For this review, take the finished solid that the model builds, in its own axes (mm). Round coordinates to 2 decimals unless told otherwise and drop trailing zeros. Loops run counter-clockwise (first coordinate to the right, second up) from the corner with the lowest first, then second, coordinate; pieces in that order, holes last. Notation, with made-up numbers: M -32.75,82 L -16.75,82 A28 ccw -16.75,111 Z; hole C 22,81.5 d3. An arc over 180 degrees is marked long. One line per question, with ' | ' between items. Start each with the question number.
1) We need section A-A (x = 25). Give the boundary of the cut face in (y, z).
2) For probe 1 along Y at (x, z) = (25, -0.95); probe 2 along X at (y, z) = (6, -1.15); probe 3 along Y at (x, z) = (-26.5, 1.4), list the stretches that pass through material, from the lowest coordinate up. Write a range as from..to.
3) For pin 1 Ø5.5 at (x, y) = (-11.42, 31.36) entering from +Z, flat-tipped, find the tip position at first contact; note if it passes through.
4) We need section B-B (z = 1.4). State how many separate pieces and enclosed holes the cut face has, and give its area (3 significant figures).
```python
from build123d import *

# Parameters (mm, degrees)
SKETCH1_W             = 330
SKETCH1_H             = 90
SKETCH1_R             = 19.05
BOSS_EXTRUDE1_DEPTH   = 2.5
M6_CLEARANCE_HOLE1_D  = 6.4
SKETCH3_R             = 8
CUT_EXTRUDE2_DEPTH    = 6
M5X0_8_TAPPED_HOLE1_D = 4.2
M5X0_8_TAPPED_HOLE3_D = 4.2
FILLET1_R             = 1.5
M3X0_5_TAPPED_HOLE1_D = 2.5


with BuildPart() as part:
    # Sketch1 → Boss-Extrude1 (new body, symmetric)
    with BuildSketch(Plane.XY):
        Rectangle(SKETCH1_W, SKETCH1_H)
        Circle(SKETCH1_R, mode=Mode.SUBTRACT)
    extrude(amount=BOSS_EXTRUDE1_DEPTH, both=True)

    # M6 Clearance Hole1 (through all)
    with Locations(Plane.XY.offset(2.5)):
        with Locations((-150, 30), (-25, 30), (-25, -30), (-150, -30)):
            m6_clearance_hole1 = Hole(M6_CLEARANCE_HOLE1_D / 2)

    # Mirror2: M6 Clearance Hole1 across plane
    add(m6_clearance_hole1.mirror(Plane(origin=(0, 0, 0), x_dir=(0, 0, 1), z_dir=(1, 0, 0))), mode=Mode.SUBTRACT)

    # Sketch3 → Cut-Extrude2 (cut, through all)
    with BuildSketch(Plane.XY.offset(2.5)):
        with Locations((-75, -0.6)):
            Circle(SKETCH3_R)
    cut_extrude2 = extrude(amount=-CUT_EXTRUDE2_DEPTH, mode=Mode.SUBTRACT)

    # M5x0.8 Tapped Hole1 (through all)
    with Locations(Plane.XY.offset(2.5)):
        with Locations((-95, -0.6), (-55, -0.6)):
            m5x0_8_tapped_hole1 = Hole(M5X0_8_TAPPED_HOLE1_D / 2)

    # Mirror1: Cut-Extrude2, M5x0.8 Tapped Hole1 across plane
    add(cut_extrude2.mirror(Plane(origin=(0, 0, 0), x_dir=(0, 0, 1), z_dir=(1, 0, 0))), mode=Mode.SUBTRACT)
    add(m5x0_8_tapped_hole1.mirror(Plane(origin=(0, 0, 0), x_dir=(0, 0, 1), z_dir=(1, 0, 0))), mode=Mode.SUBTRACT)

    # M5x0.8 Tapped Hole3 (through all)
    with Locations(Plane.XY.offset(2.5)):
        with Locations((-11.415072797, 31.362654751), (11.415072797, -31.362654751), (-31.362654751, -11.415072797), (31.362654751, 11.415072797)):
            Hole(M5X0_8_TAPPED_HOLE3_D / 2)

    # Fillet1
    fillet1_edges = [part.edges().sort_by_distance(p)[0] for p in [
        (-165, 45, 0),
        (165, 45, 0),
        (165, -45, 0),
        (-165, -45, 0),
    ]]
    fillet(fillet1_edges, radius=FILLET1_R)

    # M3x0.5 Tapped Hole1 (through all)
    with Locations(Plane.XY.offset(2.5)):
        with Locations((-50, 8), (-30, 8)):
            Hole(M3X0_5_TAPPED_HOLE1_D / 2)


solid = part.part
```
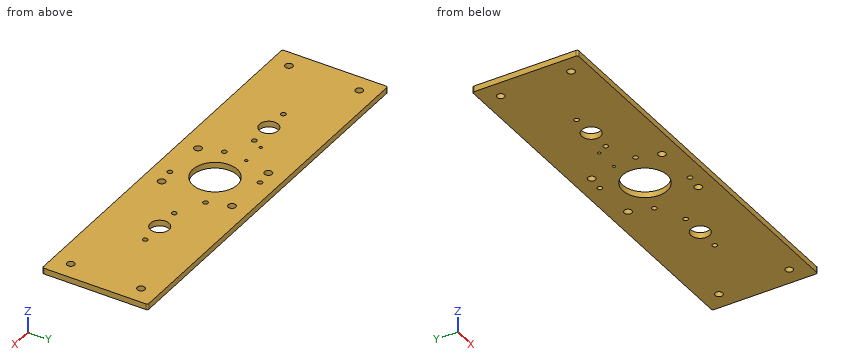
Answers below:
1) outline: M -45,-2.5 L -33.2,-2.5 L -33.2,2.5 L -45,2.5 Z; M -26.8,-2.5 L 26.8,-2.5 L 26.8,2.5 L -26.8,2.5 Z; M 33.2,-2.5 L 45,-2.5 L 45,2.5 L 33.2,2.5 Z
2) probe 1: -45..-33.2, -26.8..26.8, 33.2..45 | probe 2: -165..-79.52, -70.48..-18.08, 18.08..70.48, 79.52..165 | probe 3: -45..-32.83, -27.17..27.17, 32.83..45
3) pin 1: z = 2.5
4) separate pieces: 1 | enclosed holes: 21 | area: 27,800 mm^2
